Verification items for the finished model (mm, model axes). Face numbers are marked on the shaded views. Round coordinates to 2 decimals unless told otherwise and drop trailing zeros. Order: outer loops, then holes, each group sorted by start corner. A loop starts at its lowest first (then second) coordinate and runs counter-clockwise, first axis right, second up. Notation, with made-up numbers: (54.5, 86) -> (88.5, 86) arc R11 ccw to (88.5, 93) -> close; hole circle Ø10 at (-29.75, -24). An arc over 180 degrees is marked (long way). Return JSON: item names as keys, results as strings. Group by question number.
1) Section check D-D on z = 6.5. Enter the section's corners in (x, y), plus the area to 3 significant figures.
2) Section check A-A on z = 0. Enter the section's corners in (x, y) (3 decimals), plus the area to 3 significant figures.
3) Section check B-B on x = 5. Enter the section's corners in (y, z).
4) Draft check along Z on the marked faces 1, 2, 3 and 4. Enter one of: pulls with the +Z half, pulls with the -Z half, needs draft (parallel to the pull), parting line crosses it, or undercut.
5) Section check C-C on y = -5. Enter the section's corners in (x, z), plus the area to 3 significant figures.
6) Scan lines: L1, parallel to Y at x = 16, z = 0; L2, parallel to Y at x = 21.75, z = 1.25; L3, parallel to Z at x = 7.5, y = -1.25. Record each from-to range of solid material in increasing order.
7) Depth check by flat-ended pin: pin 1 (5 mm diameter, centred on y = -2.5, z = 0.5, fed in from +X). Enter the tip coordinate at first touch or a pass-through.
```python
from build123d import *

# Parameters (mm, degrees)
BOSS_EXTRUDE1_DEPTH                    = 25.4
TAP_DRILL_FOR_5_16_18_TAP1_D           = 6.5278
TAP_DRILL_FOR_5_16_18_TAP1_CSINK_D     = 7.7978
TAP_DRILL_FOR_5_16_18_TAP1_CSINK_ANGLE = 90


with BuildPart() as part:
    # Sketch1 → Boss-Extrude1 (new body)
    with BuildSketch(Plane(origin=(0, 0, 0), x_dir=(0, 0, -1), z_dir=(1, 0, 0))):
        Polygon((7.332348419, 0), (3.666174209, 6.35), (-3.666174209, 6.35), (-7.332348419, 0), (-3.666174209, -6.35), (3.666174209, -6.35), align=None)
    extrude(amount=BOSS_EXTRUDE1_DEPTH)

    # Tap Drill for 5/16-18 Tap1 (through all)
    with Locations(Plane(origin=(25.4, 0, 0), x_dir=(0, 0, -1), z_dir=(1, 0, 0))):
        with Locations((0, 0)):
            CounterSinkHole(TAP_DRILL_FOR_5_16_18_TAP1_D / 2, TAP_DRILL_FOR_5_16_18_TAP1_CSINK_D / 2, counter_sink_angle=TAP_DRILL_FOR_5_16_18_TAP1_CSINK_ANGLE)


solid = part.part
```
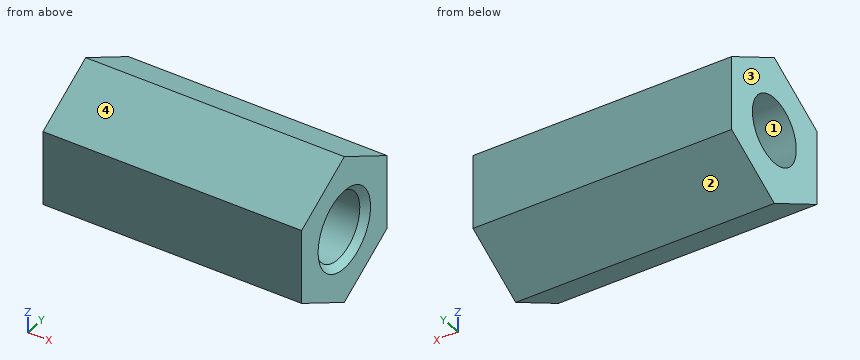
Check result:
{
 "1": {"outline": "(0, -1.44) -> (25.4, -1.44) -> (25.4, 1.44) -> (0, 1.44) -> close", "area": "73.2 mm^2"},
 "2": {"outline": "(0, -6.35) -> (25.4, -6.35) -> (25.4, -3.899) -> (24.765, -3.264) -> (0, -3.264) -> close; (0, 3.264) -> (24.765, 3.264) -> (25.4, 3.899) -> (25.4, 6.35) -> (0, 6.35) -> close", "area": "156 mm^2"},
 "3": {"outline": "(-6.35, -3.67) -> (0, -7.33) -> (6.35, -3.67) -> (6.35, 3.67) -> (0, 7.33) -> (-6.35, 3.67) -> close; hole circle Ø6.53 at (0, 0)"},
 "4": {"face 1": "undercut", "face 2": "pulls with the -Z half", "face 3": "needs draft", "face 4": "pulls with the +Z half"},
 "5": {"outline": "(0, -4.45) -> (25.4, -4.45) -> (25.4, 4.45) -> (0, 4.45) -> close", "area": "226 mm^2"},
 "6": {"L1": "-6.35 to -3.26, 3.26 to 6.35", "L2": "-6.35 to -3.02, 3.02 to 6.35", "L3": "-6.61 to -3.02, 3.02 to 6.61"},
 "7": {"pin 1": "x = 25.4"}
}
